```python
from build123d import *

# Parameters (mm, degrees)
RESSALTO_EXTRUS_O1_DEPTH = 2
FILETE1_R                = 5
ESBO_O2_R                = 4
CORTE_EXTRUS_O1_DEPTH    = 116.438914874
CORTE_EXTRUS_O2_DEPTH    = 116.438914874
RESSALTO_EXTRUS_O2_DEPTH = 4
ESBO_O5_R                = 3
CORTE_EXTRUS_O3_DEPTH    = 130.950013194
ESBO_O6_W                = 20
ESBO_O6_H                = 6
RESSALTO_EXTRUS_O3_DEPTH = 25


with BuildPart() as part:
    # Esboço1 → Ressalto-extrusão1 (new, symmetric)
    with BuildSketch(Plane.XY):
        with BuildLine():
            Line((-11.35, 0), (11.35, 0))
            Line((11.35, 0), (11.35, 26.084614768))
            ThreePointArc((11.35, 26.084614768), (11.680869588, 27.873251455), (12.62968848, 29.425165949))
            Line((12.62968848, 29.425165949), (61.077778408, 83.380928741))
            ThreePointArc((61.077778408, 83.380928741), (62.97541619, 86.484757728), (63.637155367, 90.062031103))
            Line((63.637155367, 90.062031103), (63.637155367, 96.231260639))
            Line((63.637155367, 96.231260639), (13.637155367, 96.231260639))
            Line((13.637155367, 96.231260639), (13.637155367, 88.53994255))
            ThreePointArc((13.637155367, 88.53994255), (13.380856015, 86.290432007), (12.62509583, 84.156231082))
            Line((12.62509583, 84.156231082), (-9.325880926, 39.150059113))
            ThreePointArc((-9.325880926, 39.150059113), (-10.837401296, 34.881657264), (-11.35, 30.382636177))
            Line((-11.35, 30.382636177), (-11.35, 0))
        make_face()
    extrude(amount=RESSALTO_EXTRUS_O1_DEPTH, both=True)

    # Filete1
    filete1_edges = [part.edges().sort_by_distance(p)[0] for p in [
        (11.35, 0, 0),
        (-11.35, 0, 0),
    ]]
    fillet(filete1_edges, radius=FILETE1_R)

    # Esboço2 → Corte-extrusão1 (cut, through all)
    with BuildSketch(Plane.XY.offset(2)):
        with Locations((0, 8)):
            Circle(ESBO_O2_R)
        with Locations((0, 18)):
            Circle(ESBO_O2_R)
    extrude(amount=-CORTE_EXTRUS_O1_DEPTH, mode=Mode.SUBTRACT)

    # Esboço3 → Corte-extrusão2 (cut, through all)
    with BuildSketch(Plane.XY.offset(2)):
        with BuildLine():
            Line((4.516208527, 43), (16.314765002, 43))
            ThreePointArc((16.314765002, 43), (17.944218319, 43.346935274), (19.291014218, 44.327559055))
            Line((19.291014218, 44.327559055), (27.372316137, 53.327559055))
            ThreePointArc((27.372316137, 53.327559055), (28.049131646, 57.629453317), (24.39606692, 60))
            Line((24.39606692, 60), (8.905801824, 60))
            ThreePointArc((8.905801824, 60), (6.786124767, 59.392192385), (5.310625639, 57.753484587))
            Line((5.310625639, 57.753484587), (0.921032342, 48.753484587))
            ThreePointArc((0.921032342, 48.753484587), (1.124016142, 44.880322943), (4.516208527, 43))
        make_face()
        with BuildLine():
            Line((51.333739981, 90), (23.537779481, 90))
            ThreePointArc((23.537779481, 90), (21.418102424, 89.392192385), (19.942603296, 87.753484587))
            Line((19.942603296, 87.753484587), (14.089812233, 75.753484587))
            ThreePointArc((14.089812233, 75.753484587), (14.292796034, 71.880322943), (17.684988418, 70))
            Line((17.684988418, 70), (40.558670757, 70))
            ThreePointArc((40.558670757, 70), (42.188124073, 70.346935274), (43.534919973, 71.327559055))
            Line((43.534919973, 71.327559055), (54.309989197, 83.327559055))
            ThreePointArc((54.309989197, 83.327559055), (54.986804707, 87.629453317), (51.333739981, 90))
        make_face()
    extrude(amount=-CORTE_EXTRUS_O2_DEPTH, mode=Mode.SUBTRACT)

    # Esboço4 → Ressalto-extrusão2 (add)
    with BuildSketch(Plane.XY.offset(2)):
        with BuildLine():
            Line((37.137155367, 96.231260639), (37.137155367, 103.481260639))
            ThreePointArc((37.137155367, 103.481260639), (46.887155367, 113.231260639), (56.637155367, 103.481260639))
            Line((56.637155367, 103.481260639), (56.637155367, 96.231260639))
            Line((56.637155367, 96.231260639), (37.137155367, 96.231260639))
        make_face()
    extrude(amount=-RESSALTO_EXTRUS_O2_DEPTH)

    # Esboço5 → Corte-extrusão3 (cut, through all)
    with BuildSketch(Plane.XY.offset(2)):
        with Locations((46.887155367, 103.481260639)):
            Circle(ESBO_O5_R)
    extrude(amount=-CORTE_EXTRUS_O3_DEPTH, mode=Mode.SUBTRACT)

    # Esboço6 → Ressalto-extrusão3 (add)
    with BuildSketch(Plane.XY.offset(2)):
        with Locations((23.637155367, 93.231260639)):
            Rectangle(ESBO_O6_W, ESBO_O6_H)
    extrude(amount=-RESSALTO_EXTRUS_O3_DEPTH)

    # Espelhar5: part across plane


with BuildPart() as part_1:
    add(part.part)
    add(part.part.mirror(Plane.XY.offset(-23)))


solid = part_1.part
```
Can you work these out from the model? Positions are in its coordinate system, mm. A direction names the side the tool comes from. Coordinates: 2 decimals unless noted, no trailing zeros. Order: outer loops, then holes, each group sorted by start corner. A loop starts at its lowest first (then second) coordinate and runs counter-clockwise, first axis right, second up.
1. For faces 5 (the face through (62.96, 86.44, 0.03)), 6 (the face through (26, 96.231, -23)), 7 (the face through (17.923, 43.337, -46.028)), which set-ups out of +Z, -Z, +X, -X, +Y, -Y let a thin tool reach every point of the face, with its end or its side?
2. If we section it at B-B (x = 58): Please give me the cut outline in (y, z), then the cut area to 3 significant figures.
3. I'm going to push flat-ended pins straight in: pin 1 (4.5 mm diameter, centred on x = 33.5, z = -0.5, fed in from +Y); pin 2 (8.5 mm diameter, centred on y = 94, z = -27.5, fed in from -X); pin 3 (1.2 mm diameter, centred on x = 14, z = -0.5, fed in from -Y); pin 4 (8 mm diameter, centred on y = 18.5, z = -9, fed in from -X). Where does each tip first touch, or does it pass through?
4. If we section it at A-A (y = 18): Please give me the cut outline in (x, z), then the cut area to 3 significant figures.
5. Thinking about a two-plate mould opening in X: for faces 1 (the face through (46.67, 113.23, 0.03)), 2 (the face through (46.24, 100.55, -46.03)), 3 (the face through (13.388, 86.321, 0.028)), 4 (the face through (14.26, 71.93, -46.03)), which applies, +X half, -X half, draft (parallel to the pull), parting line (faces both ways), or undercut?
6. If we section it at D-D (x = 30.5): Please give me the cut outline in (y, z).
7. I need wall thicknesses on line 1 (Z direction, x = 53, y = 75); line 2 (Y direction, x = 0, z = 0); line 3 (X direction, y = 20, z = -1). Which ranges of each line are inside material? Lowest first, please.
8. If we section it at C-C (y = 97.5): Please give me the cut outline in (x, z), then the cut area to 3 significant figures.
Entries:
1. face 5: +Z, -Z, +X, -Y
1. face 6: +Z, -Z, -X, +Y
1. face 7: +Z, -Z
2. outline: (79.95, -48) - (96.23, -48) - (96.23, -44) - (79.95, -44) - close; (79.95, -2) - (96.23, -2) - (96.23, 2) - (79.95, 2) - close
2. area: 130 mm2
3. pin 1: stops at y = 96.23
3. pin 2: stops at x = 13.64
3. pin 3: stops at y = 30.28
3. pin 4: passes through
4. outline: (-11.35, -48) - (-4, -48) - (-4, -44) - (-11.35, -44) - close; (-11.35, -2) - (-4, -2) - (-4, 2) - (-11.35, 2) - close; (4, -48) - (11.35, -48) - (11.35, -44) - (4, -44) - close; (4, -2) - (11.35, -2) - (11.35, 2) - (4, 2) - close
4. area: 118 mm2
5. face 1: parting line
5. face 2: undercut
5. face 3: -X half
5. face 4: undercut
6. outline: (49.33, -48) - (70, -48) - (70, -44) - (49.33, -44) - close; (49.33, -2) - (70, -2) - (70, 2) - (49.33, 2) - close; (90, -48) - (96.23, -48) - (96.23, 2) - (90, 2) - (90, -2) - (90.23, -2) - (90.23, -44) - (90, -44) - close
7. line 1: z = -48 to -44, -2 to 2
7. line 2: y = 0 to 4, 12 to 14, 22 to 58.27
7. line 3: x = -11.35 to -3.46, 3.46 to 11.35
8. outline: (37.14, -48) - (56.64, -48) - (56.64, -44) - (37.14, -44) - close; (37.14, -2) - (56.64, -2) - (56.64, 2) - (37.14, 2) - close
8. area: 156 mm2
